Part model, mm, in its own coordinate system. Coordinates: 2 decimals unless noted, no trailing zeros. Order: outer loops, then holes, each group sorted by start corner. A loop starts at its lowest first (then second) coordinate and runs counter-clockwise, first axis right, second up.
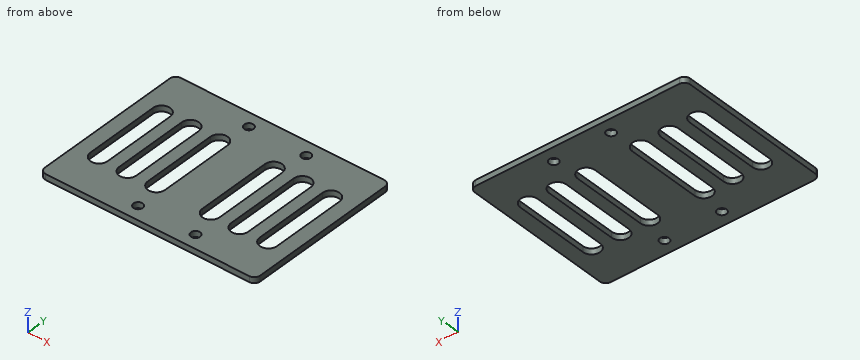
from build123d import *

# Parameters (mm, degrees)
SKETCH_1_W      = 75
SKETCH_1_H      = 56
SKETCH_1_R      = 1.6
EXTRUDE_1_DEPTH = 2
FILLET_1_R      = 2


with BuildPart() as part:
    # 草图1 → 凸台-拉伸1 (new body)
    with BuildSketch(Plane.XY):
        Rectangle(SKETCH_1_W, SKETCH_1_H)
        with Locations((12.5, 23)):
            Circle(SKETCH_1_R, mode=Mode.SUBTRACT)
        with Locations((-7.5, 23)):
            Circle(SKETCH_1_R, mode=Mode.SUBTRACT)
        with Locations(Location((-7.5, -23, 0), (0, 0, 180))):
            Circle(SKETCH_1_R, mode=Mode.SUBTRACT)
        with Locations(Location((12.5, -23, 0), (0, 0, 180))):
            Circle(SKETCH_1_R, mode=Mode.SUBTRACT)
        with BuildLine():
            Line((32.5, 13), (32.5, -13))
            ThreePointArc((32.5, -13), (29.5, -16), (26.5, -13))
            Line((26.5, -13), (26.5, 13))
            ThreePointArc((26.5, 13), (29.5, 16), (32.5, 13))
        make_face(mode=Mode.SUBTRACT)
        with BuildLine():
            Line((22.5, 13), (22.5, -13))
            ThreePointArc((22.5, -13), (19.5, -16), (16.5, -13))
            Line((16.5, -13), (16.5, 13))
            ThreePointArc((16.5, 13), (19.5, 16), (22.5, 13))
        make_face(mode=Mode.SUBTRACT)
        with BuildLine():
            Line((12.5, 13), (12.5, -13))
            ThreePointArc((12.5, -13), (9.5, -16), (6.5, -13))
            Line((6.5, -13), (6.5, 13))
            ThreePointArc((6.5, 13), (9.5, 16), (12.5, 13))
        make_face(mode=Mode.SUBTRACT)
        with BuildLine():
            Line((-12.5, 13), (-12.5, -13))
            ThreePointArc((-12.5, -13), (-9.5, -16), (-6.5, -13))
            Line((-6.5, -13), (-6.5, 13))
            ThreePointArc((-6.5, 13), (-9.5, 16), (-12.5, 13))
        make_face(mode=Mode.SUBTRACT)
        with BuildLine():
            Line((-22.5, 13), (-22.5, -13))
            ThreePointArc((-22.5, -13), (-19.5, -16), (-16.5, -13))
            Line((-16.5, -13), (-16.5, 13))
            ThreePointArc((-16.5, 13), (-19.5, 16), (-22.5, 13))
        make_face(mode=Mode.SUBTRACT)
        with BuildLine():
            Line((-32.5, 13), (-32.5, -13))
            ThreePointArc((-32.5, -13), (-29.5, -16), (-26.5, -13))
            Line((-26.5, -13), (-26.5, 13))
            ThreePointArc((-26.5, 13), (-29.5, 16), (-32.5, 13))
        make_face(mode=Mode.SUBTRACT)
    extrude(amount=EXTRUDE_1_DEPTH)

    # 圆角1
    fillet_1_edges = [part.edges().sort_by_distance(p)[0] for p in [
        (-37.5, 28, 1),
        (37.5, 28, 1),
        (37.5, -28, 1),
        (-37.5, -28, 1),
    ]]
    fillet(fillet_1_edges, radius=FILLET_1_R)


solid = part.part
Q1. Cut at D-D on z = 0.75. Count the separate pieces of the cut face and the enclosed holes in it, and give its area (3 significant figures).
Results list:
separate pieces: 1
enclosed holes: 10
area: 3,060 mm2
Q2. Cut at A-A on y = -23. Write the cut outline in (x, z).
Results list:
outline: (-37.5, 0) - (-9.1, 0) - (-9.1, 2) - (-37.5, 2) - close; (-5.9, 0) - (10.9, 0) - (10.9, 2) - (-5.9, 2) - close; (14.1, 0) - (37.5, 0) - (37.5, 2) - (14.1, 2) - close
Q3. Cut at B-B on y = 11. Write the cut outline in (x, z).
Results list:
outline: (-37.5, 0) - (-32.5, 0) - (-32.5, 2) - (-37.5, 2) - close; (-26.5, 0) - (-22.5, 0) - (-22.5, 2) - (-26.5, 2) - close; (-16.5, 0) - (-12.5, 0) - (-12.5, 2) - (-16.5, 2) - close; (-6.5, 0) - (6.5, 0) - (6.5, 2) - (-6.5, 2) - close; (12.5, 0) - (16.5, 0) - (16.5, 2) - (12.5, 2) - close; (22.5, 0) - (26.5, 0) - (26.5, 2) - (22.5, 2) - close; (32.5, 0) - (37.5, 0) - (37.5, 2) - (32.5, 2) - close
Q4. Cut at C-C on x = -29.5. Write the cut outline in (y, z), and give its area (3 significant figures).
Results list:
outline: (-28, 0) - (-16, 0) - (-16, 2) - (-28, 2) - close; (16, 0) - (28, 0) - (28, 2) - (16, 2) - close
area: 48.0 mm2
Q5. Pin check, flat tip, straight feed: pin 1 Ø5 at (x, y) = (-9.5, 10) entering from -Z. Stop position of the tip, or through.
Results list:
pin 1: passes through
Q6. Wall check: line 1 along X through (y, z) = (-23, 1.55); line 2 along Y through (x, z) = (-7.5, 1.65); line 3 along Y through (x, z) = (-30.5, 1.2). Give the ranges that are in metal, low to high.
Results list:
line 1: x = -37.5 to -9.1, -5.9 to 10.9, 14.1 to 37.5
line 2: y = -28 to -24.6, -21.4 to -15.24, 15.24 to 21.4, 24.6 to 28
line 3: y = -28 to -15.83, 15.83 to 28
